CAD build for the part. Positions are in the model's coordinates, mm. Give positions to 0.01 mm unless a question says otherwise; leave off trailing zeros. Loops run counter-clockwise (first coordinate to the right, second up) from the corner with the lowest first, then second, coordinate; pieces in that order, holes last.
Item 1: Saw through at C-C on y = 6.25. Give the cut face in (x, z).
Item 2: Probe probe 1 along X at (y, z) = (3.5, 0); probe 2 along Z at (x, y) = (0.5, 6.75); probe 3 along Z at (x, y) = (0.5, 5.75). List the from-to ranges inside material, lowest first.
Item 3: Mould opens along Z. For faces 1 (the flat face through (-2, 7, 3)), 2 (the cylindrical face through (0.406, 3.458, -3.712)), 3 (the cylindrical face through (-2.44, 3.46, -0.54)) say: released by +Z, released by -Z, zero draft, split by the parting line, or undercut.
Item 4: Saw through at A-A on x = 0. Give the number of separate pieces and of enclosed holes in the cut face, plus the area to 3 significant figures.
Item 5: Drop flat-ended pins along their axis: P1, Ø1, axis at x = -2, z = 0.5, coming from the +Y side; P2, Ø2.5, axis at x = 0, z = -5, coming from the -Y side; P3, Ø1.5, axis at x = -4.5, y = 3.5, coming from the -Z side; P4, Ø1.5, axis at y = 3.5, z = -2.5, coming from the -X side. Give the stop position or say it passes through.
from build123d import *

# Parameters (mm, degrees)
SKETCH_1_R      = 8.5
SKETCH_1_R_2    = 1.35
SKETCH_1_R_3    = 2.5
EXTRUDE_1_DEPTH = 7
CHAMFER_1_SIZE  = 0.5


with BuildPart() as part:
    # 草图1 → 凸台-拉伸1 (new body)
    with BuildSketch(Plane(origin=(0, 0, 0), x_dir=(1, 0, 0), z_dir=(0, 1, 0))):
        with Locations(Location((0, 0, 0), (0, 0, 270))):
            Circle(SKETCH_1_R)
        with Locations(Location((-5, 0, 0), (0, 0, 270))):
            Circle(SKETCH_1_R_2, mode=Mode.SUBTRACT)
        with Locations(Location((0, 5, 0), (0, 0, 270))):
            Circle(SKETCH_1_R_2, mode=Mode.SUBTRACT)
        with Locations(Location((5, 0, 0), (0, 0, 270))):
            Circle(SKETCH_1_R_2, mode=Mode.SUBTRACT)
        with Locations(Location((0, -5, 0), (0, 0, 270))):
            Circle(SKETCH_1_R_2, mode=Mode.SUBTRACT)
        with Locations(Location((0, 0, 0), (0, 0, 270))):
            Circle(SKETCH_1_R_3, mode=Mode.SUBTRACT)
    extrude(amount=EXTRUDE_1_DEPTH)

    # 倒角1
    chamfer_1_edges = [part.edges().sort_by_distance(p)[0] for p in [
        (0, 0, -6.35),
        (0, 7, -6.35),
        (5, 0, -1.35),
        (5, 7, -1.35),
        (0, 0, -8.5),
        (0, 0, 3.65),
        (0, 7, 3.65),
        (0, 7, -8.5),
        (-5, 0, -1.35),
        (-5, 7, -1.35),
        (0, 0, -2.5),
        (0, 7, -2.5),
    ]]
    chamfer(chamfer_1_edges, length=CHAMFER_1_SIZE)


solid = part.part
Results below:
1. outline: circle Ø17 at (0, 0); hole circle Ø2.7 at (-5, 0); hole circle Ø5 at (0, 0); hole circle Ø2.7 at (0, -5); hole circle Ø2.7 at (0, 5); hole circle Ø2.7 at (5, 0)
2. probe 1: x = -8.5 to -6.35, -3.65 to -2.5, 2.5 to 3.65, 6.35 to 8.5
2. probe 2: z = -8.23 to -6.52, -3.48 to -2.7, 2.7 to 3.48, 6.52 to 8.23
2. probe 3: z = -8.49 to -6.25, -3.75 to -2.45, 2.45 to 3.75, 6.25 to 8.49
3. face 1: zero draft
3. face 2: undercut
3. face 3: undercut
4. separate pieces: 4
4. enclosed holes: 0
4. area: 44.2 mm2
5. P1: stops at y = 6.56
5. P2: passes through
5. P3: stops at z = -7.63
5. P4: stops at x = -8.32
